```python
from build123d import *

# Parameters (mm, degrees)
SKETCH1_R           = 7.5
BOSS_EXTRUDE1_DEPTH = 5
SKETCH2_R           = 7.5
BOSS_EXTRUDE2_DEPTH = 1.5
BOSS_EXTRUDE3_DEPTH = 1.5
SKETCH4_W           = 5
SKETCH4_H           = 3
BOSS_EXTRUDE4_DEPTH = 6
CUT_EXTRUDE1_REACH  = 58.12
SKETCH5_W           = 1.5
SKETCH5_H           = 4.5
CUT_EXTRUDE2_REACH  = 50.936
SKETCH7_W           = 4.5
SKETCH7_H           = 1.5
CUT_EXTRUDE3_REACH  = 43.172
SKETCH8_W           = 4.5
SKETCH8_H           = 1.5
SKETCH9_W           = 3
SKETCH9_H           = 6
CUT_EXTRUDE4_DEPTH  = 3


with BuildPart() as part:
    # Sketch1 → Boss-Extrude1 (new body)
    with BuildSketch(Plane.XY):
        with BuildLine():
            Line((7.794228634, -4.5), (-1.955771366, -21.387495374))
            ThreePointArc((-1.955771366, -21.387495374), (-5.25, -24.681724008), (-9.75, -25.887495374))
            Line((-9.75, -25.887495374), (-29.25, -25.887495374))
            ThreePointArc((-29.25, -25.887495374), (-33.75, -24.681724008), (-37.044228634, -21.387495374))
            Line((-37.044228634, -21.387495374), (-46.794228634, -4.5))
            ThreePointArc((-46.794228634, -4.5), (-46.794228634, 4.5), (-39, 9))
            Line((-39, 9), (0, 9))
            ThreePointArc((0, 9), (7.794228634, 4.5), (7.794228634, -4.5))
        make_face()
        with Locations((-29.25, -16.887495374)):
            Circle(SKETCH1_R, mode=Mode.SUBTRACT)
        with Locations((-19.5, 0)):
            Circle(SKETCH1_R, mode=Mode.SUBTRACT)
        Circle(SKETCH1_R, mode=Mode.SUBTRACT)
        with Locations((-9.75, -16.887495374)):
            Circle(SKETCH1_R, mode=Mode.SUBTRACT)
        with Locations((-39, 0)):
            Circle(SKETCH1_R, mode=Mode.SUBTRACT)
    extrude(amount=BOSS_EXTRUDE1_DEPTH)

    # Sketch2 → Boss-Extrude2 (add)
    # profile 1 of 6: a face of its own
    with BuildSketch(Plane.XY.offset(5)):
        with BuildLine():
            Line((-1.955771366, -21.387495374), (7.794228634, -4.5))
            ThreePointArc((7.794228634, -4.5), (7.794228634, 4.5), (0, 9))
            Line((0, 9), (-39, 9))
            ThreePointArc((-39, 9), (-46.794228634, 4.5), (-46.794228634, -4.5))
            Line((-46.794228634, -4.5), (-37.044228634, -21.387495374))
            ThreePointArc((-37.044228634, -21.387495374), (-33.75, -24.681724008), (-29.25, -25.887495374))
            Line((-29.25, -25.887495374), (-9.75, -25.887495374))
            ThreePointArc((-9.75, -25.887495374), (-5.25, -24.681724008), (-1.955771366, -21.387495374))
        make_face()
        Circle(SKETCH2_R, mode=Mode.SUBTRACT)
        with Locations((-19.5, 0)):
            Circle(SKETCH2_R, mode=Mode.SUBTRACT)
        with Locations((-39, 0)):
            Circle(SKETCH2_R, mode=Mode.SUBTRACT)
        with Locations((-29.25, -16.887495374)):
            Circle(SKETCH2_R, mode=Mode.SUBTRACT)
        with Locations((-9.75, -16.887495374)):
            Circle(SKETCH2_R, mode=Mode.SUBTRACT)
    # profile 2 of 6: a face of its own
    with BuildSketch(Plane.XY.offset(5)):
        with Locations((-9.75, -16.887495374)):
            Circle(SKETCH2_R)
        with BuildLine():
            ThreePointArc((-13.540063509, -18.452077936), (-14.223076211, -18.635090638), (-14.040063509, -19.31810334))
            Line((-14.040063509, -19.31810334), (-9.709936491, -21.81810334))
            ThreePointArc((-9.709936491, -21.81810334), (-9.026923789, -21.635090638), (-9.209936491, -20.952077936))
            Line((-9.209936491, -20.952077936), (-13.540063509, -18.452077936))
        make_face(mode=Mode.SUBTRACT)
    # profile 3 of 6: a face of its own
    with BuildSketch(Plane.XY.offset(5)):
        Circle(SKETCH2_R)
        with BuildLine():
            ThreePointArc((-0.040063509, 4.930607966), (-0.723076211, 4.747595264), (-0.540063509, 4.064582562))
            Line((-0.540063509, 4.064582562), (3.790063509, 1.564582562))
            ThreePointArc((3.790063509, 1.564582562), (4.473076211, 1.747595264), (4.290063509, 2.430607966))
            Line((4.290063509, 2.430607966), (-0.040063509, 4.930607966))
        make_face(mode=Mode.SUBTRACT)
    # profile 4 of 6: a face of its own
    with BuildSketch(Plane.XY.offset(5)):
        with Locations((-19.5, 0)):
            Circle(SKETCH2_R)
        with BuildLine():
            ThreePointArc((-19.540063509, 4.930607966), (-20.223076211, 4.747595264), (-20.040063509, 4.064582562))
            Line((-20.040063509, 4.064582562), (-15.709936491, 1.564582562))
            ThreePointArc((-15.709936491, 1.564582562), (-15.026923789, 1.747595264), (-15.209936491, 2.430607966))
            Line((-15.209936491, 2.430607966), (-19.540063509, 4.930607966))
        make_face(mode=Mode.SUBTRACT)
    # profile 5 of 6: a face of its own
    with BuildSketch(Plane.XY.offset(5)):
        with Locations((-29.25, -16.887495374)):
            Circle(SKETCH2_R)
        with BuildLine():
            ThreePointArc((-33.040063509, -18.452077936), (-33.723076211, -18.635090638), (-33.540063509, -19.31810334))
            Line((-33.540063509, -19.31810334), (-29.209936491, -21.81810334))
            ThreePointArc((-29.209936491, -21.81810334), (-28.526923789, -21.635090638), (-28.709936491, -20.952077936))
            Line((-28.709936491, -20.952077936), (-33.040063509, -18.452077936))
        make_face(mode=Mode.SUBTRACT)
    # profile 6 of 6: a face of its own
    with BuildSketch(Plane.XY.offset(5)):
        with Locations((-39, 0)):
            Circle(SKETCH2_R)
        with BuildLine():
            ThreePointArc((-42.790063509, -1.564582562), (-43.473076211, -1.747595264), (-43.290063509, -2.430607966))
            Line((-43.290063509, -2.430607966), (-38.959936491, -4.930607966))
            ThreePointArc((-38.959936491, -4.930607966), (-38.276923789, -4.747595264), (-38.459936491, -4.064582562))
            Line((-38.459936491, -4.064582562), (-42.790063509, -1.564582562))
        make_face(mode=Mode.SUBTRACT)
        with BuildLine():
            ThreePointArc((-39.040063509, 4.930607966), (-39.723076211, 4.747595264), (-39.540063509, 4.064582562))
            Line((-39.540063509, 4.064582562), (-35.209936491, 1.564582562))
            ThreePointArc((-35.209936491, 1.564582562), (-34.526923789, 1.747595264), (-34.709936491, 2.430607966))
            Line((-34.709936491, 2.430607966), (-39.040063509, 4.930607966))
        make_face(mode=Mode.SUBTRACT)
    extrude(amount=BOSS_EXTRUDE2_DEPTH)

    # Sketch3 → Boss-Extrude3 (add)
    with BuildSketch(Plane.XY.offset(6.5)):
        with BuildLine():
            ThreePointArc((-39, 9), (-46.794228634, 4.5), (-46.794228634, -4.5))
            Line((-46.794228634, -4.5), (-46.144709581, -5.625))
            Line((-46.144709581, -5.625), (-38.985335738, 6.775399247))
            Line((-38.985335738, 6.775399247), (-33.139664262, 3.400399247))
            Line((-33.139664262, 3.400399247), (-42.247595264, -12.375))
            Line((-42.247595264, -12.375), (-37.044228634, -21.387495374))
            ThreePointArc((-37.044228634, -21.387495374), (-36.712405778, -21.918648323), (-36.344447387, -22.425438699))
            Line((-36.344447387, -22.425438699), (-34.985335738, -20.07138827))
            Line((-34.985335738, -20.07138827), (-19.610335738, 6.558892896))
            Line((-19.610335738, 6.558892896), (-13.764664262, 3.183892896))
            Line((-13.764664262, 3.183892896), (-29.139664262, -23.44638827))
            Line((-29.139664262, -23.44638827), (-30.498775911, -25.800438699))
            ThreePointArc((-30.498775911, -25.800438699), (-29.875903375, -25.865704826), (-29.25, -25.887495374))
            Line((-29.25, -25.887495374), (-18.84326674, -25.887495374))
            Line((-18.84326674, -25.887495374), (-15.485335738, -20.07138827))
            Line((-15.485335738, -20.07138827), (-0.110335738, 6.558892896))
            Line((-0.110335738, 6.558892896), (5.735335738, 3.183892896))
            Line((5.735335738, 3.183892896), (-9.639664262, -23.44638827))
            Line((-9.639664262, -23.44638827), (-11.049038106, -25.887495374))
            Line((-11.049038106, -25.887495374), (-9.75, -25.887495374))
            ThreePointArc((-9.75, -25.887495374), (-5.25, -24.681724008), (-1.955771366, -21.387495374))
            Line((-1.955771366, -21.387495374), (7.794228634, -4.5))
            ThreePointArc((7.794228634, -4.5), (7.794228634, 4.5), (0, 9))
            Line((0, 9), (-39, 9))
        make_face()
    extrude(amount=BOSS_EXTRUDE3_DEPTH)

    # Sketch4 → Boss-Extrude4 (add)
    with BuildSketch(Plane(origin=(0, 0, 0), x_dir=(-1, 0, 0), z_dir=(0, 0, -1))):
        Polygon((40.669228634, -15.108811196), (43.169228634, -10.778684177), (40.571152423, -9.278684177), (38.071152423, -13.608811196), align=None)
        with Locations((19.5, -24.387495374)):
            Rectangle(SKETCH4_W, SKETCH4_H)
        Polygon((-4.169228634, -10.778684177), (-1.669228634, -15.108811196), (0.928847577, -13.608811196), (-1.571152423, -9.278684177), align=None)
        with Locations((9.75, 7.5)):
            Rectangle(SKETCH4_W, SKETCH4_H)
        with Locations((29.25, 7.5)):
            Rectangle(SKETCH4_W, SKETCH4_H)
    extrude(amount=BOSS_EXTRUDE4_DEPTH)

    # Sketch5 → Cut-Extrude1 (cut, up to next)
    with BuildSketch(Plane(origin=(-6.125, 10.608811196, 0), x_dir=(0.8660254037844386, 0.5000000000000001, 0), z_dir=(-0.5000000000000001, 0.8660254037844386, 0)), mode=Mode.PRIVATE) as cut_extrude1_sk1:
        with Locations((-42.024990748, 2.25)):
            Rectangle(SKETCH5_W, SKETCH5_H)
    cut_extrude1_tool1 = extrude(cut_extrude1_sk1.sketch, amount=-CUT_EXTRUDE1_REACH, mode=Mode.PRIVATE) & part.part
    # Sketch5 → Cut-Extrude1 (cut, up to next)
    with BuildSketch(Plane(origin=(-6.125, 10.608811196, 0), x_dir=(0.8660254037844386, 0.5000000000000001, 0), z_dir=(-0.5000000000000001, 0.8660254037844386, 0)), mode=Mode.PRIVATE) as cut_extrude1_sk2:
        Polygon((-42.774990748, 6), (-42.774990748, 4.5), (-41.274990748, 6), align=None)
    cut_extrude1_tool2 = extrude(cut_extrude1_sk2.sketch, amount=-CUT_EXTRUDE1_REACH, mode=Mode.PRIVATE) & part.part
    cut_extrude1_1 = cut_extrude1_tool1.solids().sort_by_distance((-42.51971, -10.403684, -2.25))[0]
    add(cut_extrude1_1, mode=Mode.SUBTRACT)
    cut_extrude1_2 = cut_extrude1_tool2.solids().sort_by_distance((-42.736216, -10.528684, -5.5))[0]
    add(cut_extrude1_2, mode=Mode.SUBTRACT)
    cut_extrude1 = cut_extrude1_1 + cut_extrude1_2  # Cut-Extrude1 as one shape, for the pattern or mirror that repeats it

    # Sketch7 → Cut-Extrude2 (cut, up to next)
    with BuildSketch(Plane.ZY.offset(31.75), mode=Mode.PRIVATE) as cut_extrude2_sk1:
        with Locations((-2.25, 8.25)):
            Rectangle(SKETCH7_W, SKETCH7_H)
    cut_extrude2_tool1 = extrude(cut_extrude2_sk1.sketch, amount=-CUT_EXTRUDE2_REACH, mode=Mode.PRIVATE) & part.part
    # Sketch7 → Cut-Extrude2 (cut, up to next)
    with BuildSketch(Plane.ZY.offset(31.75), mode=Mode.PRIVATE) as cut_extrude2_sk2:
        Polygon((-6, 7.5), (-4.5, 9), (-6, 9), align=None)
    cut_extrude2_tool2 = extrude(cut_extrude2_sk2.sketch, amount=-CUT_EXTRUDE2_REACH, mode=Mode.PRIVATE) & part.part
    cut_extrude2_1 = cut_extrude2_tool1.solids().sort_by_distance((-31.75, 8.25, -2.25))[0]
    add(cut_extrude2_1, mode=Mode.SUBTRACT)
    cut_extrude2_2 = cut_extrude2_tool2.solids().sort_by_distance((-31.75, 8.5, -5.5))[0]
    add(cut_extrude2_2, mode=Mode.SUBTRACT)
    cut_extrude2 = cut_extrude2_1 + cut_extrude2_2  # Cut-Extrude2 as one shape, for the pattern or mirror that repeats it

    # Mirror1: Cut-Extrude1, Cut-Extrude2 across plane
    add(cut_extrude1.mirror(Plane(origin=(-19.5, 0, 0), x_dir=(0, 0, 1), z_dir=(1, 0, 0))), mode=Mode.SUBTRACT)
    add(cut_extrude2.mirror(Plane(origin=(-19.5, 0, 0), x_dir=(0, 0, 1), z_dir=(1, 0, 0))), mode=Mode.SUBTRACT)

    # Sketch8 → Cut-Extrude3 (cut, up to next)
    with BuildSketch(Plane.ZY.offset(22), mode=Mode.PRIVATE) as cut_extrude3_sk1:
        Polygon((-6, -25.887495374), (-4.5, -25.887495374), (-6, -24.387495374), align=None)
    cut_extrude3_tool1 = extrude(cut_extrude3_sk1.sketch, amount=-CUT_EXTRUDE3_REACH, mode=Mode.PRIVATE) & part.part
    # Sketch8 → Cut-Extrude3 (cut, up to next)
    with BuildSketch(Plane.ZY.offset(22), mode=Mode.PRIVATE) as cut_extrude3_sk2:
        with Locations((-2.25, -25.137495374)):
            Rectangle(SKETCH8_W, SKETCH8_H)
    cut_extrude3_tool2 = extrude(cut_extrude3_sk2.sketch, amount=-CUT_EXTRUDE3_REACH, mode=Mode.PRIVATE) & part.part
    add(cut_extrude3_tool1.solids().sort_by_distance((-22, -25.387495, -5.5))[0], mode=Mode.SUBTRACT)
    add(cut_extrude3_tool2.solids().sort_by_distance((-22, -25.137495, -2.25))[0], mode=Mode.SUBTRACT)

    # Sketch9 → Cut-Extrude4 (cut)
    with BuildSketch(Plane.XY.offset(8)):
        with Locations((-29.25, 6)):
            Rectangle(SKETCH9_W, SKETCH9_H)
        with Locations((-9.75, 6)):
            Rectangle(SKETCH9_W, SKETCH9_H)
    extrude(amount=-CUT_EXTRUDE4_DEPTH, mode=Mode.SUBTRACT)


solid = part.part
```
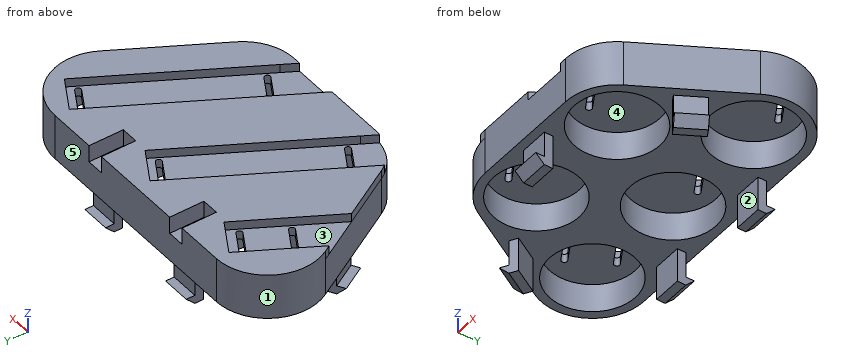
Here's how the part is built. I have some questions about the finished solid (model axes, mm). Face numbers are marked on the shaded views. A direction names the side the tool comes from. Coordinates: 2 decimals unless noted, no trailing zeros. Order: outer loops, then holes, each group sorted by start corner. A loop starts at its lowest first (then second) coordinate and runs counter-clockwise, first axis right, second up.
1) Imagine slicing it at C-C on y = 0. List the corners of the cut face in (x, z) for me, and give its area (3 significant figures).
2) Will these pins go through, and if not, where does the flat tip stop? pin 1 (4 mm diameter, centred on y = -19, z = 4, fed in from -X); pin 2 (2.5 mm diameter, centred on y = 7.5, z = -2, fed in from +X); pin 3 (1.5 mm diameter, centred on y = 7, z = 6, fed in from -X).
3) Imagine slicing it at A-A on z = -1.75. List the corners of the cut face in (x, y) for me.
4) Imagine slicing it at B-B on z = 3.5. List the corners of the cut face in (x, y) for me, and give its area (3 significant figures).
5) I need wall thicknesses on line 1 (Y direction, x = -29.25, z = 1.2); line 2 (Y direction, x = -4.5, z = 4.75); line 3 (X direction, y = -13, z = 6.75). Which ranges of each line are inside material? Lowest first, please.
6) Which directions (+Z, -Z, +X, -X, +Y, -Y) give clear straight access to the entire face, cutting with the end or side of a thin tool? Please do the marked faces 1, 2, 3, 4 and 5.
Response values:
1. outline: (-48, 0) - (-46.5, 0) - (-46.5, 5) - (-31.5, 5) - (-31.5, 0) - (-27, 0) - (-27, 5) - (-12, 5) - (-12, 0) - (-7.5, 0) - (-7.5, 5) - (7.5, 5) - (7.5, 0) - (9, 0) - (9, 8) - (3.9, 8) - (3.9, 6.5) - (-3.9, 6.5) - (-3.9, 8) - (-15.6, 8) - (-15.6, 6.5) - (-23.4, 6.5) - (-23.4, 8) - (-35.1, 8) - (-35.1, 6.5) - (-42.9, 6.5) - (-42.9, 8) - (-48, 8) - close
1. area: 196 mm2
2. pin 1: stops at x = -39.58
2. pin 2: stops at x = -7.25
2. pin 3: stops at x = -45.48
3. outline: (-41.87, -10.03) - (-39.37, -14.36) - (-38.07, -13.61) - (-40.57, -9.28) - close; (-31.75, 6) - (-26.75, 6) - (-26.75, 7.5) - (-31.75, 7.5) - close; (-22, -24.39) - (-17, -24.39) - (-17, -22.89) - (-22, -22.89) - close; (-12.25, 6) - (-7.25, 6) - (-7.25, 7.5) - (-12.25, 7.5) - close; (-0.93, -13.61) - (0.37, -14.36) - (2.87, -10.03) - (1.57, -9.28) - close
4. outline: (-46.79, -4.5) - (-37.04, -21.39) arc R9 ccw to (-29.25, -25.89) - (-9.75, -25.89) arc R9 ccw to (-1.96, -21.39) - (7.79, -4.5) arc R9 ccw to (0, 9) - (-39, 9) arc R9 ccw to start; hole circle Ø15 at (-39, 0); hole circle Ø15 at (-29.25, -16.89); hole circle Ø15 at (-19.5, 0); hole circle Ø15 at (-9.75, -16.89); hole circle Ø15 at (0, 0)
4. area: 742 mm2
5. line 1: y = -25.89 to -24.39, -9.39 to 9
5. line 2: y = -24.2 to -22.24, -11.53 to -6, 6 to 9
5. line 3: x = -41.89 to -30.9, -23.11 to -11.4, -3.61 to 2.89
6. face 1: +Z, -Z, -X
6. face 2: -Z, +X, -X, -Y
6. face 3: +Z
6. face 4: -Z
6. face 5: +Z, -Z, +X, -X, +Y
